Could you check a few things on this drawing? It's one solid part, dimensions in mm from its lowest x, y, z. A direction names the side the tool comes from. Give positions to 0.01 mm unless a question says otherwise; leave off trailing zeros. Loops run counter-clockwise (first coordinate to the right, second up) from the corner with the lowest first, then second, coordinate; pieces in that order, holes last. Notation, with made-up numbers: (11, 78.5) - (51, 78.5) arc R36 cw to (51, 112.5) - close; hole circle Ø10 at (-7, 41). An arc over 180 degrees is marked (long way). Write each question's results on one line, items separated by ' | '. Start each with the question number.
(1) If we mould it in two halves opening along Z, with no side actions, what happens to the marked faces 1, 2 and 3? For each: released by +Z, released by -Z, zero draft, split by the parting line, or undercut.
(2) Suppose I cut it at A-A (z = 20). Please give me the cut outline in (x, y) (1 decimal).
(3) For pin 1 (17 mm diameter, centred on x = 17.5, z = 16.5, fed in from +Y); pin 2 (3 mm diameter, centred on y = 2.5, z = 13, fed in from -X) (1 decimal), each with a flat end and sliding along its axis, tell me the tip position at first contact or that it passes through.
(4) Suppose I cut it at B-B (x = 20). Please give me the cut outline in (y, z) (1 decimal).
(5) Suppose I cut it at C-C (y = 0.5). Please give me the cut outline in (x, z) (1 decimal).
(6) Suppose I cut it at D-D (y = 3.5). Please give me the cut outline in (x, z) (1 decimal), and give its area (3 significant figures).
(7) On a 3-axis mill with a long thin cutter (end or side, diameter ignored), from which of +Z, -Z, +X, -X, +Y, -Y can I reach the whole of each face in a straight line? I mean the marked faces 4, 5 and 6. Say none if no direction works.
(8) I need wall thicknesses on line 1 (Y direction, x = 21.5, z = 21); line 2 (Z direction, x = 8.5, y = 1); line 3 (Z direction, x = 2, y = 6) (1 decimal). Which ranges of each line are inside material? Lowest first, please.
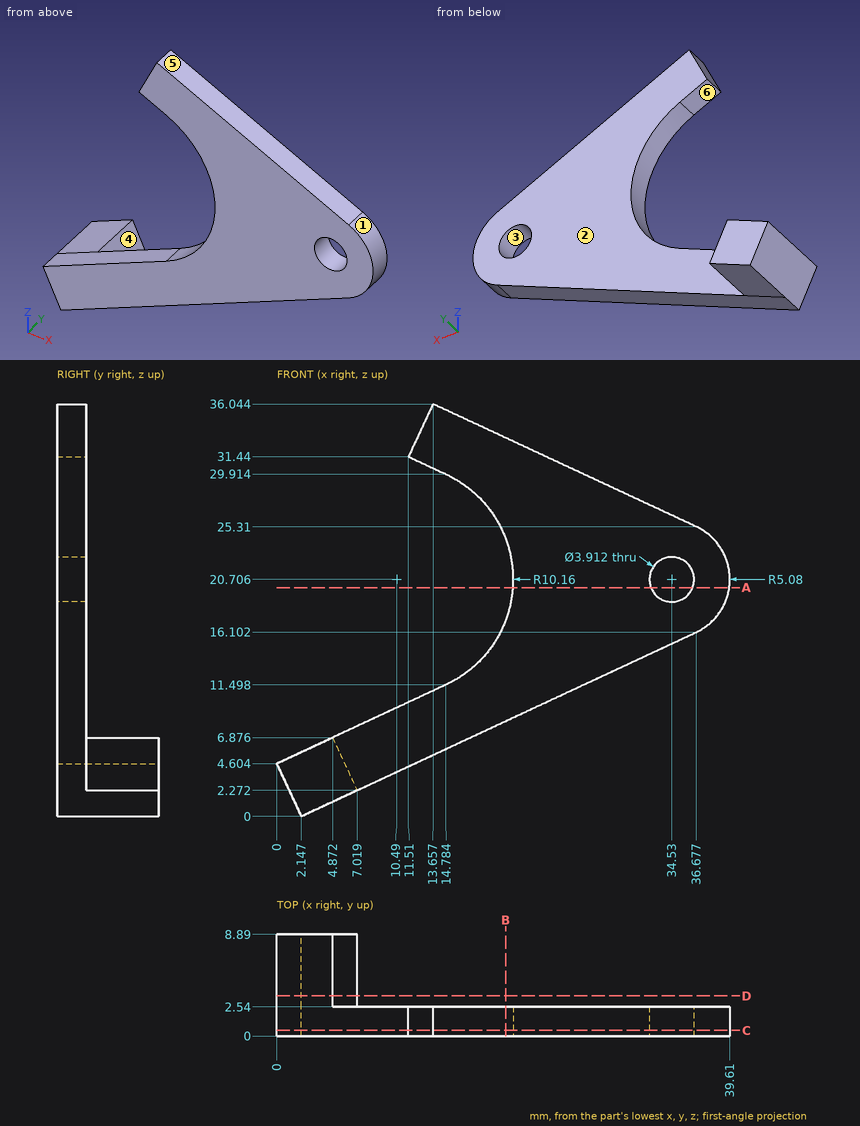
Output values:
1) face 1: split by the parting line | face 2: zero draft | face 3: undercut
2) outline: (20.6, 0) - (32.7, 0) - (32.7, 2.5) - (20.6, 2.5) - close; (36.4, 0) - (39.6, 0) - (39.6, 2.5) - (36.4, 2.5) - close
3) pin 1: y = 2.54 | pin 2: x = 14.8
4) outline: (0, 8.3) - (2.5, 8.3) - (2.5, 17.1) - (0, 17.1) - close; (0, 24.3) - (2.5, 24.3) - (2.5, 33.1) - (0, 33.1) - close
5) outline: (0, 4.6) - (2.1, 0) - (36.7, 16.1) arc R5.1 ccw to (36.7, 25.3) - (13.7, 36) - (11.5, 31.4) - (14.8, 29.9) arc R10.2 cw to (14.8, 11.5) - close; hole circle Ø3.9 at (34.5, 20.7)
6) outline: (0, 4.6) - (2.1, 0) - (7, 2.3) - (4.9, 6.9) - close | area: 27.3 mm2
7) face 4: +Z, +X, +Y | face 5: +Z, +X, +Y, -Y | face 6: -X, +Y, -Y
8) line 1: 0 to 2.54 | line 2: 2.96 to 8.57 | line 3: 0.3 to 5.5
